Geometry check sheet. Reference: drawing and pictorial views, mm from the part's lowest x, y, z. A direction names the side the tool comes from. Coordinates: 2 decimals unless noted, no trailing zeros. Loops run counter-clockwise (first coordinate to the right, second up) from the corner with the lowest first, then second, coordinate; pieces in that order, holes last. Notation, with made-up numbers: (84.25, 85.5) -> (119.25, 85.5) arc R21 ccw to (119.25, 94.5) -> close; hole circle Ø4 at (61.25, 87). An arc over 180 degrees is marked (long way). Answer as a JSON object with one key per item and string values.
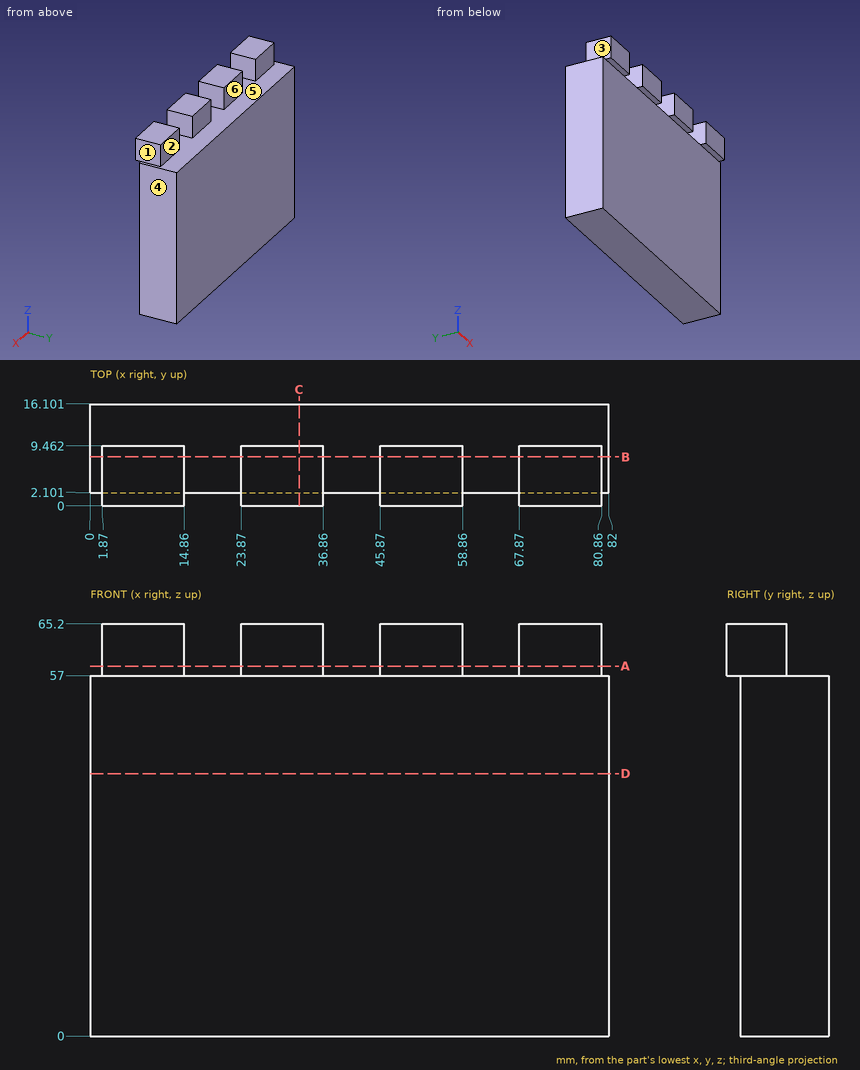
1. Section check C-C, the plane x = 33. Record the boundary of the cut face in (y, z).
Evaluation:
{"outline": "(0, 57) -> (2.1, 57) -> (2.1, 0) -> (16.1, 0) -> (16.1, 57) -> (9.46, 57) -> (9.46, 65.2) -> (0, 65.2) -> close"}
2. Section check B-B, the plane y = 7.75. Record the boundary of the cut face in (x, z).
Evaluation:
{"outline": "(0, 0) -> (82, 0) -> (82, 57) -> (80.86, 57) -> (80.86, 65.2) -> (67.87, 65.2) -> (67.87, 57) -> (58.86, 57) -> (58.86, 65.2) -> (45.87, 65.2) -> (45.87, 57) -> (36.86, 57) -> (36.86, 65.2) -> (23.87, 65.2) -> (23.87, 57) -> (14.86, 57) -> (14.86, 65.2) -> (1.87, 65.2) -> (1.87, 57) -> (0, 57) -> close"}
3. Mould release check, pull along X, two halves, no side actions. Record for the marked faces 4, 5 and 6: released by +X, released by -X, zero draft, split by the parting line, or undercut.
Evaluation:
{"face 4": "released by +X", "face 5": "undercut", "face 6": "zero draft"}
4. Depth check by flat-ended pin: P1, Ø2.5, axis at y = 3, z = 59.5, coming from the +X side; P2, Ø1.1, axis at x = 9, y = 1, coming from the -Z side; P3, Ø4, axis at x = 52.5, z = 62, coming from the +Y side. Enter the tip coordinate at first touch or a pass-through.
Evaluation:
{"P1": "stops at x = 80.86", "P2": "stops at z = 57", "P3": "stops at y = 9.46"}
5. Section check A-A, the plane z = 58.5. Record the boundary of the cut face in (x, y).
Evaluation:
{"outline": "(1.87, 0) -> (14.86, 0) -> (14.86, 9.46) -> (1.87, 9.46) -> close; (23.87, 0) -> (36.86, 0) -> (36.86, 9.46) -> (23.87, 9.46) -> close; (45.87, 0) -> (58.86, 0) -> (58.86, 9.46) -> (45.87, 9.46) -> close; (67.87, 0) -> (80.86, 0) -> (80.86, 9.46) -> (67.87, 9.46) -> close"}
6. Thickness scan on probe 1 along Z at (x, y) = (47.5, 11.5); probe 2 along Y at (x, z) = (30.5, 11.5); probe 3 along Y at (x, z) = (5, 60). Record the ranges inside material, lowest first. Write a range as from..to.
Evaluation:
{"probe 1": "z = 0..57", "probe 2": "y = 2.1..16.1", "probe 3": "y = 0..9.46"}
7. Tool access check on the marked faces 1, 2 and 3. Record the directions out of +Z, -Z, +X, -X, +Y, -Y that give a thin tool (end or side, any length) a straight path to the whole face; none if there is none.
Evaluation:
{"face 1": "+Z, +X, +Y, -Y", "face 2": "+Z, +X, -X, +Y", "face 3": "+Z, -X, +Y, -Y"}
8. Section check D-D, the plane z = 41.5. Record the boundary of the cut face in (x, y).
Evaluation:
{"outline": "(0, 2.1) -> (82, 2.1) -> (82, 16.1) -> (0, 16.1) -> close"}
